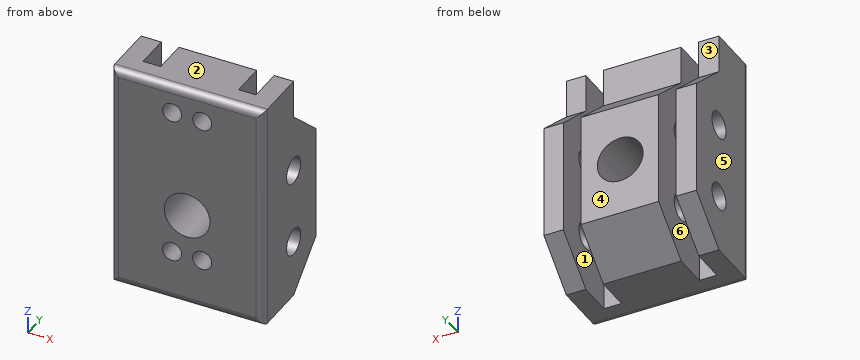
```python
from build123d import *

# Parameters (mm, degrees)
SKETCH1_W           = 63.5
SKETCH1_H           = 6.35
BOSS_EXTRUDE1_DEPTH = 50.8
BOSS_EXTRUDE2_DEPTH = 50.8
SKETCH10_W          = 5.842
SKETCH10_H          = 25.629031657
CUT_EXTRUDE1_DEPTH  = 88.854357354
LPATTERN3_COUNT     = 2
LPATTERN3_PITCH     = 31.75
SKETCH11_R          = 4.445
CUT_EXTRUDE2_DEPTH  = 88.854357354
BOSS_EXTRUDE3_DEPTH = 12.7
SKETCH23_R          = 7.62
CUT_EXTRUDE6_DEPTH  = 88.854357354
FILLET2_R           = 2.54
SKETCH24_R          = 3.175
CUT_EXTRUDE7_DEPTH  = 10


with BuildPart() as part:
    # Sketch1 → Boss-Extrude1 (new body)
    with BuildSketch(Plane(origin=(0, 0, 0), x_dir=(0, 0, -1), z_dir=(1, 0, 0))):
        with Locations((31.75, 3.175)):
            Rectangle(SKETCH1_W, SKETCH1_H)
    extrude(amount=-BOSS_EXTRUDE1_DEPTH)

    # Sketch2 → Boss-Extrude2 (add)
    with BuildSketch(Plane(origin=(0, 0, 0), x_dir=(0, 0, -1), z_dir=(1, 0, 0))):
        Polygon((0, 6.35), (0, 19.05), (12.7, 33.249031657), (50.8, 33.249031657), (63.5, 19.05), (63.5, 6.35), align=None)
    extrude(amount=-BOSS_EXTRUDE2_DEPTH)

    # Sketch10 → Cut-Extrude1 (cut, through all)
    with BuildSketch(Plane(origin=(0, 0, -63.5), x_dir=(-1, 0, 0), z_dir=(0, 0, -1))):
        with Locations((9.398, 20.434515829)):
            Rectangle(SKETCH10_W, SKETCH10_H)
    cut_extrude1 = extrude(amount=-CUT_EXTRUDE1_DEPTH, mode=Mode.SUBTRACT)

    # LPattern3: Cut-Extrude1 ×2
    with Locations(*[(-i * LPATTERN3_PITCH, 0, 0) for i in range(1, LPATTERN3_COUNT)]):
        add(cut_extrude1, mode=Mode.SUBTRACT)

    # Sketch11 → Cut-Extrude2 (cut, through all)
    with BuildSketch(Plane(origin=(0, 0, 0), x_dir=(0, 0, -1), z_dir=(1, 0, 0))):
        with Locations((19.05, 19.05)):
            Circle(SKETCH11_R)
        with Locations((44.45, 19.05)):
            Circle(SKETCH11_R)
    extrude(amount=-CUT_EXTRUDE2_DEPTH, mode=Mode.SUBTRACT)

    # Sketch22 → Boss-Extrude3 (add)
    with BuildSketch(Plane.XY):
        Polygon((0, 0), (-50.8, 0), (-50.8, 7.62), (-50.8, 19.05), (-44.069, 19.05), (-44.069, 7.62), (-38.227, 7.62), (-38.227, 19.05), (-12.319, 19.05), (-12.319, 7.62), (-6.477, 7.62), (-6.477, 19.05), (0, 19.05), (0, 7.62), align=None)
    extrude(amount=BOSS_EXTRUDE3_DEPTH)

    # Sketch23 → Cut-Extrude6 (cut, through all)
    with BuildSketch(Plane(origin=(0, 33.249031657, 0), x_dir=(1, 0, 0), z_dir=(0, 1, 0))):
        with Locations(Location((-25.4, 31.75, 0), (0, 0, 270))):
            Circle(SKETCH23_R)
    extrude(amount=-CUT_EXTRUDE6_DEPTH, mode=Mode.SUBTRACT)

    # Fillet2
    fillet2_edges = [part.edges().sort_by_distance(p)[0] for p in [
        (-25.4, 0, 12.7),
        (0, 0, -25.4),
        (-50.8, 0, -25.4),
        (-25.4, 0, -63.5),
    ]]
    fillet(fillet2_edges, radius=FILLET2_R)

    # Sketch24 → Cut-Extrude7 (cut)
    with BuildSketch(Plane.XZ):
        with Locations(Location((-30.4, -46.15, 0), (0, 0, 270))):
            Circle(SKETCH24_R)
        with Locations(Location((-20.4, -46.15, 0), (0, 0, 270))):
            Circle(SKETCH24_R)
        with Locations(Location((-20.4, 3.35, 0), (0, 0, 270))):
            Circle(SKETCH24_R)
        with Locations(Location((-30.4, 3.35, 0), (0, 0, 270))):
            Circle(SKETCH24_R)
    extrude(amount=-CUT_EXTRUDE7_DEPTH, mode=Mode.SUBTRACT)


solid = part.part
```
Source: CAD feature listing. Evaluate the final solid. Frame: model axes, mm. Face numbers are marked on the shaded views. A direction names the side the tool comes from. Round coordinates to 2 decimals unless told otherwise and drop trailing zeros. Loops run counter-clockwise (first coordinate to the right, second up) from the corner with the lowest first, then second, coordinate; pieces in that order, holes last.
(1) Access query for the marked faces 1, 2 and 3. Directions: +Z, -Z, +X, -X, +Y, -Y. A direction counts if a zero-diameter tool reaches every point of the face in a straight line with its end or side. Return the directions, or none.
From the geometry:
face 1: +Z, -Z, +Y
face 2: +Z, +X, -X, +Y, -Y
face 3: +Z, +X, -X, +Y
(2) Contact query for flat-ended pins moving along their axis: pin 1 Ø5.5 at (y, z) = (19.05, -19.05) entering from +X; pin 2 Ø2 at (x, z) = (-37, 0) entering from +Y; pin 3 Ø3 at (x, y) = (-18.5, 26) entering from -Z; pin 4 Ø2 at (x, z) = (-48, 6) entering from +Y. Output: stop coordinate, or through.
From the geometry:
pin 1: passes through
pin 2: stops at y = 20.17
pin 3: stops at z = -58.63
pin 4: stops at y = 19.05
(3) Section query C-C (z = -31.75). Output: boundary loops of the cut face in (x, y), and give its area (3 significant figures).
From the geometry:
outline: (-50.8, 2.54) arc R2.54 ccw to (-48.26, 0) - (-33.02, 0) - (-33.02, 33.25) - (-38.23, 33.25) - (-38.23, 7.62) - (-44.07, 7.62) - (-44.07, 33.25) - (-50.8, 33.25) - close; (-17.78, 0) - (-2.54, 0) arc R2.54 ccw to (0, 2.54) - (0, 33.25) - (-6.48, 33.25) - (-6.48, 7.62) - (-12.32, 7.62) - (-12.32, 33.25) - (-17.78, 33.25) - close
area: 880 mm2
(4) Pull-direction query (X, two-part tool) for the marked faces 4, 5 and 6; classes: +X half, -X half, draft (parallel to the pull), parting line (faces both ways), or undercut.
From the geometry:
face 4: draft
face 5: -X half
face 6: undercut
(5) Section query B-B (y = 29). Output: boundary loops of the cut face in (x, z).
From the geometry:
outline: (-50.8, -54.6) - (-44.07, -54.6) - (-44.07, -8.9) - (-50.8, -8.9) - close; (-38.23, -54.6) - (-12.32, -54.6) - (-12.32, -8.9) - (-38.23, -8.9) - close; (-6.48, -54.6) - (0, -54.6) - (0, -8.9) - (-6.48, -8.9) - close; hole circle Ø15.24 at (-25.4, -31.75)
(6) Section query A-A (x = -25.4). Output: boundary loops of the cut face in (y, z) (3 decimals), and give its area (3 significant figures).
From the geometry:
outline: (0, -60.96) arc R2.54 ccw to (2.54, -63.5) - (19.05, -63.5) - (33.249, -50.8) - (33.249, -39.37) - (0, -39.37) - close; (0, -24.13) - (33.249, -24.13) - (33.249, -12.7) - (19.05, 0) - (19.05, 12.7) - (2.54, 12.7) arc R2.54 ccw to (0, 10.16) - close; hole circle Ø8.89 at (19.05, -44.45); hole circle Ø8.89 at (19.05, -19.05)
area: 1,540 mm2
(7) Material intervals for probe 1 along X at (y, z) = (18.5, -7); probe 2 along Z at (x, y) = (-37.5, 19); probe 3 along X at (y, z) = (7, 3.35) (3 decimals), sorted ascending.
From the geometry:
probe 1: x = -50.8 to -44.07, -38.23 to -12.32, -6.48 to 0
probe 2: z = -63.5 to -48.89, -40.01 to -23.49, -14.61 to 12.7
probe 3: x = -50.8 to -33.575, -27.225 to -23.575, -17.225 to 0
(8) Section query D-D (z = -42). Output: boundary loops of the cut face in (x, y), and give its area (3 significant figures).
From the geometry:
outline: (-50.8, 2.54) arc R2.54 ccw to (-48.26, 0) - (-2.54, 0) arc R2.54 ccw to (0, 2.54) - (0, 15.34) - (-6.48, 15.34) - (-6.48, 7.62) - (-12.32, 7.62) - (-12.32, 15.34) - (-38.23, 15.34) - (-38.23, 7.62) - (-44.07, 7.62) - (-44.07, 15.34) - (-50.8, 15.34) - close; (-50.8, 22.76) - (-44.07, 22.76) - (-44.07, 33.25) - (-50.8, 33.25) - close; (-38.23, 22.76) - (-12.32, 22.76) - (-12.32, 33.25) - (-38.23, 33.25) - close; (-6.48, 22.76) - (0, 22.76) - (0, 33.25) - (-6.48, 33.25) - close
area: 1,100 mm2
